The listing builds one solid part. Answer for the finished solid, in the listing's coordinates (mm). A direction names the side the tool comes from. Round coordinates to 2 decimals unless told otherwise and drop trailing zeros. Write item = value, one per line. Start each with the question number.
1) Given pin 1 Ø6.5 at (y, z) = (-26, 17.5) entering from +X; pin 2 Ø6 at (y, z) = (-55.5, 39.5) entering from -X; pin 3 Ø7.5 at (y, z) = (-8, 37.5) entering from -X; pin 4 Ø1.5 at (x, y) = (-36, 55) entering from -Z (3 decimals), each flat-ended and moving along its own axis, determine where each tip first touches the part or whether it passes through.
2) For a pull along Y with two mould halves and no side action, classify faces 3 (the flat face through (-57, -49, 12.7)), 4 (the flat face through (43.2, 55.4, 0)), 5 (the cylindrical face through (0.2, -76.2, 12.5)) as released by +Y, released by -Y, zero draft, split by the parting line, or undercut.
3) Section A-A, the plane z = 7.5 is taken. Give the number of separate pieces and of enclosed holes in the cut face, and give its area (3 significant figures).
4) A tool of negligible diameter and unlimited length cuts with its end or side. For faces 1 (the cylindrical face through (-10.98, 68.98, 19.14)), 2 (the cylindrical face through (20.14, 73.93, 12.52)), from which of +Z, -Z, +X, -X, +Y, -Y can it reach the whole face along a straight path? Write none if from no direction.
5) Straight lines are drawn through the part: line 1 along X through (y, z) = (57.15, 3.5); line 2 along Y through (x, z) = (37, 19.5) (3 decimals). For each, find the intervals that lie inside material, in ascending order.
from build123d import *

# Parameters (mm, degrees)
BASE_EXTRUDE_DEPTH      = 25.4
BOSS_EXTRUDE1_DEPTH     = 25.4
CUT_EXTRUDE1_DEPTH      = 25.4
CUT_EXTRUDE1_DRAFT      = -7
CUT_EXTRUDE3_DEPTH      = 12.7
BOSS_EXTRUDE2_REACH     = 121.475
SKETCH6_W               = 25.134955719
SKETCH6_H               = 12.7
CIRPATTERN1_COUNT       = 4
CUT_EXTRUDE4_DEPTH      = 12.7
CUT_EXTRUDE4_DEPTH_BACK = 123.803155497
SKETCH7_R               = 6.35
CHAMFER1_SIZE           = 1.27
CUT_EXTRUDE5_START      = -3.175
SKETCH17_R              = 69.85
SKETCH17_R_2            = 50.8
CUT_EXTRUDE5_DEPTH      = 3.175
SKETCH28_R              = 8.0645
CUT_EXTRUDE6_DEPTH      = 120.474537036


with BuildPart() as part:
    # Sketch1 → Base-Extrude (new body)
    with BuildSketch(Plane.XY):
        with BuildLine():
            Line((-50.575996254, 81.684515988), (-23.24962088, 74.362435774))
            ThreePointArc((-23.24962088, 74.362435774), (-20.186868638, 73.931673761), (-17.110816292, 74.25402323))
            ThreePointArc((-17.110816292, 74.25402323), (0, 76.2), (17.110816292, 74.25402323))
            ThreePointArc((17.110816292, 74.25402323), (20.186868638, 73.931673761), (23.24962088, 74.362435774))
            Line((23.24962088, 74.362435774), (50.575996254, 81.684515988))
            ThreePointArc((50.575996254, 81.684515988), (75.110512242, 75.110512242), (81.684515988, 50.575996254))
            Line((81.684515988, 50.575996254), (74.362435774, 23.24962088))
            ThreePointArc((74.362435774, 23.24962088), (73.931673761, 20.186868638), (74.25402323, 17.110816292))
            ThreePointArc((74.25402323, 17.110816292), (76.2, 0), (74.25402323, -17.110816292))
            ThreePointArc((74.25402323, -17.110816292), (73.931673761, -20.186868638), (74.362435774, -23.24962088))
            Line((74.362435774, -23.24962088), (81.684515988, -50.575996254))
            ThreePointArc((81.684515988, -50.575996254), (75.110512242, -75.110512242), (50.575996254, -81.684515988))
            Line((50.575996254, -81.684515988), (23.24962088, -74.362435774))
            ThreePointArc((23.24962088, -74.362435774), (20.186868638, -73.931673761), (17.110816292, -74.25402323))
            ThreePointArc((17.110816292, -74.25402323), (0, -76.2), (-17.110816292, -74.25402323))
            ThreePointArc((-17.110816292, -74.25402323), (-20.186868638, -73.931673761), (-23.24962088, -74.362435774))
            Line((-23.24962088, -74.362435774), (-50.575996254, -81.684515988))
            ThreePointArc((-50.575996254, -81.684515988), (-75.110512242, -75.110512242), (-81.684515988, -50.575996254))
            Line((-81.684515988, -50.575996254), (-74.362435774, -23.24962088))
            ThreePointArc((-74.362435774, -23.24962088), (-73.931673761, -20.186868638), (-74.25402323, -17.110816292))
            ThreePointArc((-74.25402323, -17.110816292), (-76.2, 0), (-74.25402323, 17.110816292))
            ThreePointArc((-74.25402323, 17.110816292), (-73.931673761, 20.186868638), (-74.362435774, 23.24962088))
            Line((-74.362435774, 23.24962088), (-81.684515988, 50.575996254))
            ThreePointArc((-81.684515988, 50.575996254), (-75.110512242, 75.110512242), (-50.575996254, 81.684515988))
        make_face()
    extrude(amount=BASE_EXTRUDE_DEPTH)

    # Sketch2 → Boss-Extrude1 (add)
    with BuildSketch(Plane.XY.offset(25.4)):
        with BuildLine():
            Line((-38.1, 50.8), (38.1, 50.8))
            ThreePointArc((38.1, 50.8), (47.080256121, 47.080256121), (50.8, 38.1))
            Line((50.8, 38.1), (50.8, -38.1))
            ThreePointArc((50.8, -38.1), (47.080256121, -47.080256121), (38.1, -50.8))
            Line((38.1, -50.8), (-38.1, -50.8))
            ThreePointArc((-38.1, -50.8), (-47.080256121, -47.080256121), (-50.8, -38.1))
            Line((-50.8, -38.1), (-50.8, 38.1))
            ThreePointArc((-50.8, 38.1), (-47.080256121, 47.080256121), (-38.1, 50.8))
        make_face()
    extrude(amount=BOSS_EXTRUDE1_DEPTH)


with BuildPart() as cut_extrude1_tool:
    # Sketch3 → Cut-Extrude1 (with draft: the straight prism first)
    with BuildSketch(Plane.XY.offset(50.8)):
        with BuildLine():
            Line((-44.45, 38.1), (-44.45, -38.1))
            ThreePointArc((-44.45, -38.1), (-42.590128061, -42.590128061), (-38.1, -44.45))
            Line((-38.1, -44.45), (38.1, -44.45))
            ThreePointArc((38.1, -44.45), (42.590128061, -42.590128061), (44.45, -38.1))
            Line((44.45, -38.1), (44.45, 38.1))
            ThreePointArc((44.45, 38.1), (42.590128061, 42.590128061), (38.1, 44.45))
            Line((38.1, 44.45), (-38.1, 44.45))
            ThreePointArc((-38.1, 44.45), (-42.590128061, 42.590128061), (-44.45, 38.1))
        make_face()
    extrude(amount=-CUT_EXTRUDE1_DEPTH)
    # Cut-Extrude1: the draft: its side faces are tilted about the plane it starts from
    cut_extrude1_sides = [cut_extrude1_tool.faces().sort_by_distance(p)[0] for p in [
        (-42.590128061, 42.590128061, 38.1),
        (-44.45, 0, 38.1),
        (-42.590128061, -42.590128061, 38.1),
        (0, -44.45, 38.1),
        (42.590128061, -42.590128061, 38.1),
        (44.45, 0, 38.1),
        (42.590128061, 42.590128061, 38.1),
        (0, 44.45, 38.1),
    ]]
    draft(cut_extrude1_sides, Plane.XY.offset(50.8), CUT_EXTRUDE1_DRAFT)


with BuildPart() as part_1:
    add(part.part)

    # Cut-Extrude1: cut by cut_extrude1_tool
    add(cut_extrude1_tool.part, mode=Mode.SUBTRACT)

    # Sketch5 → Cut-Extrude3 (cut)
    with BuildSketch(Plane.XY.offset(25.4)):
        with BuildLine():
            Line((-75.550886991, 52.219497191), (-68.228806777, 24.893121817))
            ThreePointArc((-68.228806777, 24.893121817), (-67.582663757, 20.298993453), (-68.066187961, 15.684914935))
            ThreePointArc((-68.066187961, 15.684914935), (-69.85, 0), (-68.066187961, -15.684914935))
            ThreePointArc((-68.066187961, -15.684914935), (-67.582663757, -20.298993453), (-68.228806777, -24.893121817))
            Line((-68.228806777, -24.893121817), (-75.550886991, -52.219497191))
            ThreePointArc((-75.550886991, -52.219497191), (-70.620384182, -70.620384182), (-52.219497191, -75.550886991))
            Line((-52.219497191, -75.550886991), (-24.893121817, -68.228806777))
            ThreePointArc((-24.893121817, -68.228806777), (-20.298993453, -67.582663757), (-15.684914935, -68.066187961))
            ThreePointArc((-15.684914935, -68.066187961), (0, -69.85), (15.684914935, -68.066187961))
            ThreePointArc((15.684914935, -68.066187961), (20.298993453, -67.582663757), (24.893121817, -68.228806777))
            Line((24.893121817, -68.228806777), (52.219497191, -75.550886991))
            ThreePointArc((52.219497191, -75.550886991), (70.620384182, -70.620384182), (75.550886991, -52.219497191))
            Line((75.550886991, -52.219497191), (68.228806777, -24.893121817))
            ThreePointArc((68.228806777, -24.893121817), (67.582663757, -20.298993453), (68.066187961, -15.684914935))
            ThreePointArc((68.066187961, -15.684914935), (69.85, 0), (68.066187961, 15.684914935))
            ThreePointArc((68.066187961, 15.684914935), (67.582663757, 20.298993453), (68.228806777, 24.893121817))
            Line((68.228806777, 24.893121817), (75.550886991, 52.219497191))
            ThreePointArc((75.550886991, 52.219497191), (70.620384182, 70.620384182), (52.219497191, 75.550886991))
            Line((52.219497191, 75.550886991), (24.893121817, 68.228806777))
            ThreePointArc((24.893121817, 68.228806777), (20.298993453, 67.582663757), (15.684914935, 68.066187961))
            ThreePointArc((15.684914935, 68.066187961), (0, 69.85), (-15.684914935, 68.066187961))
            ThreePointArc((-15.684914935, 68.066187961), (-20.298993453, 67.582663757), (-24.893121817, 68.228806777))
            Line((-24.893121817, 68.228806777), (-52.219497191, 75.550886991))
            ThreePointArc((-52.219497191, 75.550886991), (-70.620384182, 70.620384182), (-75.550886991, 52.219497191))
        make_face()
        with BuildLine():
            Line((-53.975, 38.1), (-53.975, -38.1))
            ThreePointArc((-53.975, -38.1), (-49.325320151, -49.325320151), (-38.1, -53.975))
            Line((-38.1, -53.975), (38.1, -53.975))
            ThreePointArc((38.1, -53.975), (49.325320151, -49.325320151), (53.975, -38.1))
            Line((53.975, -38.1), (53.975, 38.1))
            ThreePointArc((53.975, 38.1), (49.325320151, 49.325320151), (38.1, 53.975))
            Line((38.1, 53.975), (-38.1, 53.975))
            ThreePointArc((-38.1, 53.975), (-49.325320151, 49.325320151), (-53.975, 38.1))
        make_face(mode=Mode.SUBTRACT)
    extrude(amount=-CUT_EXTRUDE3_DEPTH, mode=Mode.SUBTRACT)

    # Sketch6 → Boss-Extrude2 (add, up to next)
    with BuildSketch(Plane.XY.offset(25.4), mode=Mode.PRIVATE) as boss_extrude2_sk1:
        with Locations((63.367477859, 0)):
            Rectangle(SKETCH6_W, SKETCH6_H)
    boss_extrude2_tool1 = extrude(boss_extrude2_sk1.sketch, amount=-BOSS_EXTRUDE2_REACH, mode=Mode.PRIVATE) - part_1.part
    boss_extrude2 = boss_extrude2_tool1.solids().sort_by_distance((63.367478, 0, 25.4))[0]
    add(boss_extrude2)

    # CirPattern1: Boss-Extrude2 ×4 about axis
    cirpattern1_axis = Axis((0, 0, -50), (0, 0, 1))
    for i in range(1, CIRPATTERN1_COUNT):
        add(boss_extrude2.rotate(cirpattern1_axis, i * 360 / CIRPATTERN1_COUNT))

    # Sketch7 → Cut-Extrude4 (cut, two sides: drawn at the far end of the back side and taken through both)
    with BuildSketch(Plane.XY.offset(12.7).offset(-CUT_EXTRUDE4_DEPTH_BACK)):
        with Locations((57.15, 57.15)):
            Circle(SKETCH7_R)
        with Locations((-57.15, 57.15)):
            Circle(SKETCH7_R)
        with Locations((-57.15, -57.15)):
            Circle(SKETCH7_R)
        with Locations((57.15, -57.15)):
            Circle(SKETCH7_R)
    extrude(amount=CUT_EXTRUDE4_DEPTH + CUT_EXTRUDE4_DEPTH_BACK, mode=Mode.SUBTRACT)

    # Chamfer1
    chamfer1_edges = [part_1.edges().sort_by_distance(p)[0] for p in [
        (50.8, -57.15, 0),
        (-63.5, -57.15, 0),
        (50.8, 57.15, 0),
        (-63.5, 57.15, 0),
        (50.8, -57.15, 12.7),
        (-63.5, -57.15, 12.7),
        (50.8, 57.15, 12.7),
        (-63.5, 57.15, 12.7),
    ]]
    chamfer(chamfer1_edges, length=CHAMFER1_SIZE)

    # Sketch17 → Cut-Extrude5 (cut)
    with BuildSketch(Plane(origin=(0, 0, 0), x_dir=(-1, 0, 0), z_dir=(0, 0, -1)).offset(CUT_EXTRUDE5_START)):
        Circle(SKETCH17_R)
        Circle(SKETCH17_R_2, mode=Mode.SUBTRACT)
    extrude(amount=CUT_EXTRUDE5_DEPTH, mode=Mode.SUBTRACT)

    # Sketch28 → Cut-Extrude6 (cut, through all)
    with BuildSketch(Plane.XY.offset(25.4)):
        Circle(SKETCH28_R)
    extrude(amount=-CUT_EXTRUDE6_DEPTH, mode=Mode.SUBTRACT)


solid = part_1.part
Geometry check:
q1.pin_1 = 75.97
q1.pin_2 = through
q1.pin_3 = -50.8
q1.pin_4 = 3.175
q2.face_3 = undercut
q2.face_4 = zero draft
q2.face_5 = released by -Y
q3.separate_pieces = 1
q3.enclosed_holes = 5
q3.area = 23,600 mm2
q4.face_1 = +Z
q4.face_2 = +Z, -Z, +Y
q5.line_1 = -82.55 to -63.5, -50.8 to 50.8, 63.5 to 82.55
q5.line_2 = -78.047 to -71.473, -53.975 to 53.975, 71.473 to 78.047
